Verification items for this drawing (mm, ordinates from the low corner). A direction names the side the tool comes from. Coordinates: 2 decimals unless noted, no trailing zeros. Loops run counter-clockwise (first coordinate to the right, second up) from the corner with the lowest first, then second, coordinate; pieces in that order, holes last. Notation, with made-up numbers: M -40,-16.75 L -2,-16.75 A19 cw -2,-1.75 Z; hole C 79,87.25 d2. An arc over 180 degrees is marked long. One line per question, with ' | ' between items. Start each with the question number.
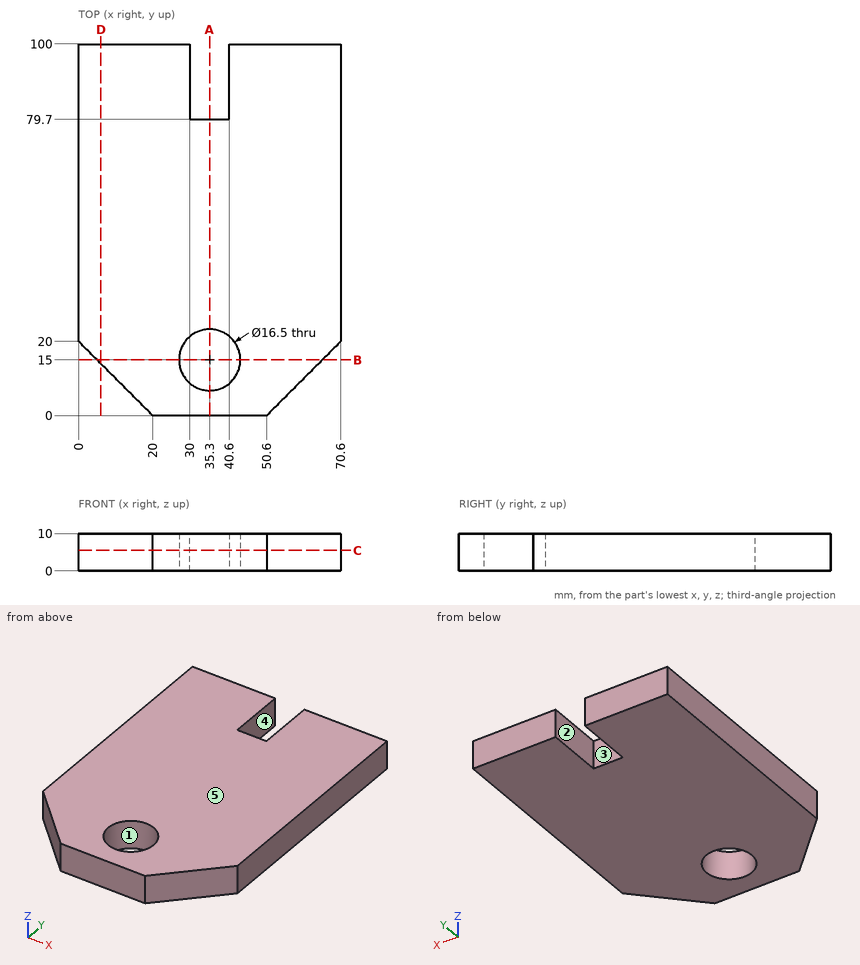
1. Draft check along Y on the marked faces 1, 2 and 3. Enter one of: +Y half, -Y half, draft (parallel to the pull), parting line (faces both ways), or undercut.
2. Depth check by flat-ended pin: pin 1 Ø4 at (y, z) = (13.5, 3) entering from -X. Enter the tip coordinate at first touch or a pass-through.
3. Sectioned sample at A-A (x = 35.3). Record the cut outline in (y, z).
4. Sectioned sample at D-D (x = 6). Record the cut outline in (y, z).
5. Sectioned sample at B-B (y = 15). Record the cut outline in (x, z).
6. Thickness scan on line 1 (X direction, y = 95, z = 8.75); line 2 (Y direction, x = 35.3, z = 3.5); line 3 (X direction, y = 15, z = 4.25). Record the ranges inside material, lowest first.
7. Tool access check on the marked faces 4 and 5. Record the directions out of +Z, -Z, +X, -X, +Y, -Y that give a thin tool (end or side, any length) a straight path to the whole face; none if there is none.
8. Sectioned sample at C-C (z = 5.5). Record the cut outline in (x, y), and give its area (3 significant figures).
Result:
1) face 1: undercut | face 2: draft | face 3: +Y half
2) pin 1: stops at x = 4.5
3) outline: M 0,0 L 6.75,0 L 6.75,10 L 0,10 Z; M 23.25,0 L 79.7,0 L 79.7,10 L 23.25,10 Z
4) outline: M 14,0 L 100,0 L 100,10 L 14,10 Z
5) outline: M 5,0 L 27.05,0 L 27.05,10 L 5,10 Z; M 43.55,0 L 65.6,0 L 65.6,10 L 43.55,10 Z
6) line 1: x = 0 to 30, 40.6 to 70.6 | line 2: y = 0 to 6.75, 23.25 to 79.7 | line 3: x = 5 to 27.05, 43.55 to 65.6
7) face 4: +Z, -Z, +Y | face 5: +Z, +X, -X, +Y, -Y
8) outline: M 0,20 L 20,0 L 50.6,0 L 70.6,20 L 70.6,100 L 40.6,100 L 40.6,79.7 L 30,79.7 L 30,100 L 0,100 Z; hole C 35.3,15 d16.5 | area: 6,230 mm2
